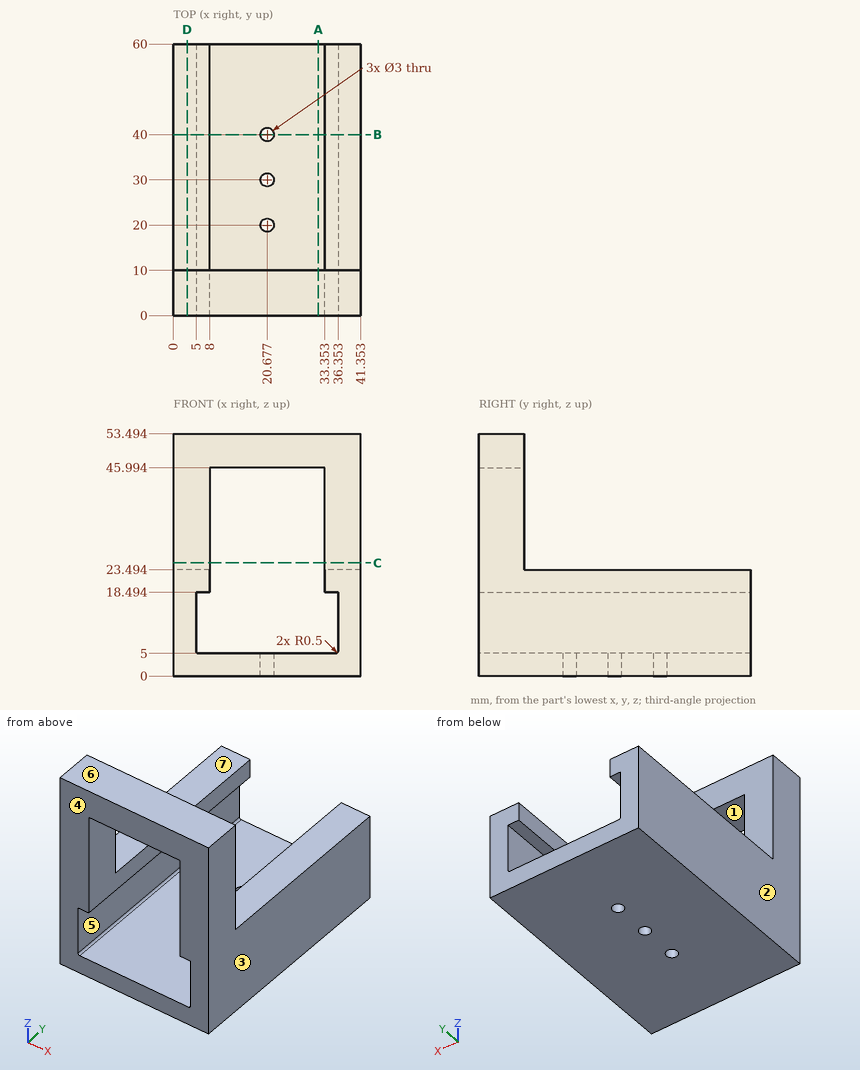
Geometry: see drawing. Coordinates: mm, zero at the bounding-box minimum. A direction names the side the tool comes from. Give positions to 0.01 mm unless a question says otherwise; leave off trailing zeros. Write each loop counter-clockwise with the first axis right and the second up, starting at its lowest first coordinate (ties: lowest second). Pieces come first, ordered by that corner, then holes. Notation, with made-up numbers: M -2,4.5 L 41,4.5 A20 ccw 41,9.5 Z; hole C 21,64.5 d10. An arc over 180 degrees is marked long. Answer in a Markdown table with one row per item. Add a question column.
(1) Mould query, pull axis X, two halves, no side actions, for the marked faces 1, 2, 3 and 4. Classes: +X half, -X half, draft (parallel to the pull), parting line (faces both ways), or undercut.
(2) Reachability of the marked faces 5, 6 and 7 from +Z, -Z, +X, -X, +Y, -Y: full face, straight path, thin tool, end or side. Return the list, or none.
(3) Section D-D on x = 3. Return loops of the section in (y, z).
(4) Section A-A on x = 32. Return loops of the section in (y, z).
(5) Ray query, line 1 (Z direction, x = 35.5, y = 49); line 2 (X direction, y = 49, z = 7.5); line 3 (Z direction, x = 31.5, y = 51). Return the intervals inside material, ascending.
(6) First-contact query: pin 1 (8 mm diameter, centred on x = 34.5, z = 31, fed in from +Y); pin 2 (4 mm diameter, centred on x = 20.68, y = 40, fed in from +Z); pin 3 (2.5 mm diameter, centred on x = 38, y = 23.5, fed in from +Z); pin 4 (1.5 mm diameter, centred on x = 31.5, z = 25.5, fed in from -Y) (1 decimal). Flat tips, straight axial feed; report the tip coordinate or a pass-through.
(7) Section C-C on z = 25. Return loops of the section in (x, y), and give its area (3 significant figures).
(8) Section B-B on y = 40. Return loops of the section in (x, z), and give its area (3 significant figures).
Result set:
| question | item | result |
|---|---|---|
| 1 | face 1 | undercut |
| 1 | face 2 | -X half |
| 1 | face 3 | +X half |
| 1 | face 4 | draft |
| 2 | face 5 | +Y, -Y |
| 2 | face 6 | +Z, +X, -X, +Y, -Y |
| 2 | face 7 | +Z, +X, -X, +Y |
| 3 | outline | M 0,0 L 60,0 L 60,23.49 L 10,23.49 L 10,53.49 L 0,53.49 Z |
| 4 | outline | M 0,0 L 60,0 L 60,5 L 0,5 Z; M 0,45.99 L 10,45.99 L 10,53.49 L 0,53.49 Z |
| 5 | line 1 | z = 0 to 5, 18.49 to 23.49 |
| 5 | line 2 | x = 0 to 5, 36.35 to 41.35 |
| 5 | line 3 | z = 0 to 5 |
| 6 | pin 1 | stops at y = 10 |
| 6 | pin 2 | stops at z = 5 |
| 6 | pin 3 | stops at z = 23.49 |
| 6 | pin 4 | passes through |
| 7 | outline | M 0,0 L 8,0 L 8,10 L 0,10 Z; M 33.35,0 L 41.35,0 L 41.35,10 L 33.35,10 Z |
| 7 | area | 160 mm^2 |
| 8 | outline | M 0,0 L 19.18,0 L 19.18,5 L 5.5,5 A0.5 cw 5,5.5 L 5,18.49 L 8,18.49 L 8,23.49 L 0,23.49 Z; M 22.18,0 L 41.35,0 L 41.35,23.49 L 33.35,23.49 L 33.35,18.49 L 36.35,18.49 L 36.35,5.5 A0.5 cw 35.85,5 L 22.18,5 Z |
| 8 | area | 407 mm^2 |
